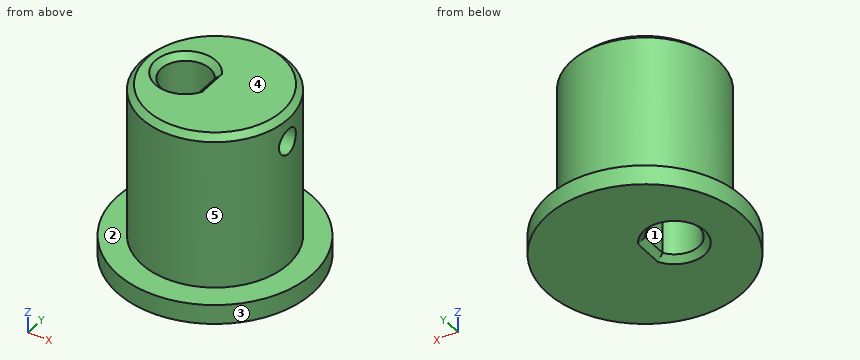
```python
from build123d import *

# Parameters (mm, degrees)
SKETCH_R        = 7.5
PAD_DEPTH       = 16
SKETCH001_R     = 10
PAD001_DEPTH    = 2
SKETCH002_R     = 1.3
POCKET_DEPTH    = 13.001
POCKET001_DEPTH = 18.001
CHAMFER_SIZE    = 0.6


with BuildPart() as part:
    # Sketch → Pad (new body)
    with BuildSketch(Plane.XY):
        with Locations((3, 0)):
            Circle(SKETCH_R)
    extrude(amount=PAD_DEPTH)

    # Sketch001 (on Face2 of Pad) → Pad001 (join)
    with BuildSketch(Plane(origin=(0, 0, 0), x_dir=(1, 0, 0), z_dir=(0, 0, -1))):
        with Locations((3, 0)):
            Circle(SKETCH001_R)
    extrude(amount=PAD001_DEPTH)

    # Sketch002 → Pocket (cut, through all)
    with BuildSketch(Plane.YZ):
        with Locations((0, 13)):
            Circle(SKETCH002_R)
    extrude(amount=POCKET_DEPTH, mode=Mode.SUBTRACT)

    # Sketch003 (on Face6 of Pocket) → Pocket001 (cut, through all)
    with BuildSketch(Plane.XY.offset(16)):
        with BuildLine():
            ThreePointArc((2.1, 1.356466), (-2.5, 0), (2.1, -1.356466))
            Line((2.1, -1.356466), (2.1, 1.356466))
        make_face()
    extrude(amount=-POCKET001_DEPTH, mode=Mode.SUBTRACT)

    # Chamfer
    chamfer_edges = [part.edges().sort_by_distance(p)[0] for p in [
        (-4.5, 0, 16),
        (2.1, 0, 16),
        (-2.5, 0, 16),
        (-2.5, 0, -2),
        (2.1, 0, -2),
    ]]
    chamfer(chamfer_edges, length=CHAMFER_SIZE)


solid = part.part
```
Input: part model. Units: mm. Frame: model coordinates. Face numbers are marked on the shaded views. A direction names the side the tool comes from. Coordinates: 2 decimals unless noted, no trailing zeros. Loops run counter-clockwise (first coordinate to the right, second up) from the corner with the lowest first, then second, coordinate; pieces in that order, holes last. Notation, with made-up numbers: M 16.25,1.5 L 71.25,1.5 A24 cw 71.25,23.5 Z; hole C -20.5,-10 d9. An arc over 180 degrees is marked long. Answer in a Markdown table with one row per item.
1. Draft query along X for the marked faces 1, 2 and 3. Return one class per face: pulls with the +X half, pulls with the -X half, needs draft (parallel to the pull), parting line crosses it, or undercut.
Response:
| item | result |
|---|---|
| face 1 | undercut |
| face 2 | needs draft |
| face 3 | parting line crosses it |
2. Reachability of the marked faces 4 and 5 from +Z, -Z, +X, -X, +Y, -Y: full face, straight path, thin tool, end or side. Return the list, or none.
Response:
| item | result |
|---|---|
| face 4 | +Z, +X, -X, +Y, -Y |
| face 5 | +Z |
3. First-contact query: pin 1 (1.6 mm diameter, centred on y = 0, z = 13, fed in from -X); pin 2 (1 mm diameter, centred on y = 2.5, z = 1.5, fed in from -X); pin 3 (5 mm diameter, centred on y = 2.5, z = 14, fed in from +X). Flat tips, straight axial feed; report the tip coordinate or a pass-through.
Response:
| item | result |
|---|---|
| pin 1 | stops at x = -4.5 |
| pin 2 | stops at x = -4.23 |
| pin 3 | stops at x = 10.5 |
4. Section C-C, the plane z = 5.5. Output: boundary loops of the cut face in (x, y).
Response:
| item | result |
|---|---|
| outline | C 3,0 d15; hole M 2.1,-1.36 L 2.1,1.36 A2.5 ccw long Z |
5. Material intervals for line 1 (Z direction, x = 6.75, y = 0); line 2 (X direction, y = 0.25, z = -0.5); line 3 (Z direction, x = -0.25, y = -8.5), sorted ascending.
Response:
| item | result |
|---|---|
| line 1 | z = -2 to 11.7, 14.3 to 16 |
| line 2 | x = -7 to -2.49, 2.1 to 13 |
| line 3 | z = -2 to 0 |
6. Section A-A, the plane y = 0. Output: boundary loops of the cut face in (x, z).
Response:
| item | result |
|---|---|
| outline | M -7,-2 L -3.1,-2 L -2.5,-1.4 L -2.5,15.4 L -3.1,16 L -3.9,16 L -4.5,15.4 L -4.5,0 L -7,0 Z; M 2.1,-1.4 L 2.7,-2 L 13,-2 L 13,0 L 10.5,0 L 10.5,11.7 L 2.1,11.7 Z; M 2.1,14.3 L 10.5,14.3 L 10.5,15.4 L 9.9,16 L 2.7,16 L 2.1,15.4 Z |
7. Section D-D, the plane z = 13. Output: boundary loops of the cut face in (x, y), then the cut area to 3 significant figures.
Response:
| item | result |
|---|---|
| outline | M 2.1,-1.36 A2.5 cw long 2.1,1.36 L 2.1,1.3 L 10.39,1.3 A7.5 ccw long 10.39,-1.3 L 2.1,-1.3 Z |
| area | 136 mm2 |
8. Section B-B, the plane x = 3. Output: boundary loops of the cut face in (y, z), then the cut area to 3 significant figures.
Response:
| item | result |
|---|---|
| outline | M -10,-2 L 10,-2 L 10,0 L 7.5,0 L 7.5,15.4 L 6.9,16 L -6.9,16 L -7.5,15.4 L -7.5,0 L -10,0 Z; hole C 0,13 d2.6 |
| area | 274 mm2 |
